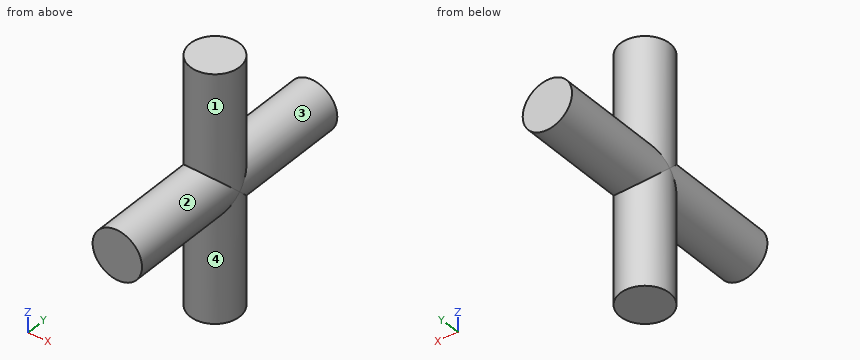
```python
from build123d import *

# Parameters (mm, degrees)
SKETCH2_R           = 5
BOSS_EXTRUDE1_DEPTH = 50
SKETCH5_R           = 5
BOSS_EXTRUDE2_DEPTH = 50


with BuildPart() as part:
    # Sketch2 → Boss-Extrude1 (new body)
    with BuildSketch(Plane.XY):
        Circle(SKETCH2_R)
    extrude(amount=BOSS_EXTRUDE1_DEPTH)

    # Sketch5 → Boss-Extrude2 (add)
    with BuildSketch(Plane(origin=(0, 25, 0), x_dir=(1, 0, 0), z_dir=(0, 1, 0))):
        with Locations((0, -25)):
            Circle(SKETCH5_R)
    extrude(amount=-BOSS_EXTRUDE2_DEPTH)


solid = part.part
```
The listing builds one solid part. Answer for the finished solid, in the listing's coordinates (mm). Face numbers are marked on the shaded views. A direction names the side the tool comes from. Give positions to 0.01 mm unless a question says otherwise; leave off trailing zeros. Loops run counter-clockwise (first coordinate to the right, second up) from the corner with the lowest first, then second, coordinate; pieces in that order, holes last. Notation, with made-up numbers: (52, 55) - (107, 55) arc R21 ccw to (107, 77) - close; hole circle Ø1 at (71, -13.5). An arc over 180 degrees is marked (long way). Return JSON: item names as keys, results as strings. Group by question number.
1. Find section C-C (x = -4). Write down the section's boundary in (y, z).
2. Find section A-A (x = 0). Write down the section's boundary in (y, z), then the cut area to 3 significant figures.
3. Find section B-B (y = 2). Write down the section's boundary in (x, z), then the cut area to 3 significant figures.
4. Straight lines are drawn through the part: line 1 (Y direction, x = -0.25, z = 39); line 2 (Y direction, x = 4, z = 38.5); line 3 (X direction, y = -4.5, z = 44). For each, find the intervals that lie inside material, in ascending order. Write a range as [from, to].
5. Which of the six approach directions +Z, -Z, +X, -X, +Y, -Y give full straight-line access (tool end or side, diameter ignored) to the marked faces 1, 2, 3 and 4?
6. Given pin 1 Ø6 at (x, y) = (-2, 12) entering from +Z; pin 2 Ø4 at (x, y) = (3, 12) entering from -Z; pin 3 Ø8 at (y, z) = (-17, 17.5) entering from +X, each flat-ended and moving along its own axis, determine where each tip first touches the part or whether it passes through.
7. Find section D-D (z = 35). Write down the section's boundary in (x, y).
Verdict:
{
 "1": {"outline": "(-25, 22) - (-3, 22) - (-3, 0) - (3, 0) - (3, 22) - (25, 22) - (25, 28) - (3, 28) - (3, 50) - (-3, 50) - (-3, 28) - (-25, 28) - close"},
 "2": {"outline": "(-25, 20) - (-5, 20) - (-5, 0) - (5, 0) - (5, 20) - (25, 20) - (25, 30) - (5, 30) - (5, 50) - (-5, 50) - (-5, 30) - (-25, 30) - close", "area": "900 mm^2"},
 "3": {"outline": "(-4.58, 0) - (4.58, 0) - (4.58, 23) arc R5 ccw to (4.58, 27) - (4.58, 50) - (-4.58, 50) - (-4.58, 27) arc R5 ccw to (-4.58, 23) - close", "area": "461 mm^2"},
 "4": {"line 1": "y = [-4.99, 4.99]", "line 2": "y = [-3, 3]", "line 3": "x = [-2.18, 2.18]"},
 "5": {"face 1": "+Z", "face 2": "-Y", "face 3": "+Y", "face 4": "-Z"},
 "6": {"pin 1": "stops at z = 30", "pin 2": "stops at z = 20.1", "pin 3": "stops at x = 3.57"},
 "7": {"outline": "circle Ø10 at (0, 0)"}
}
